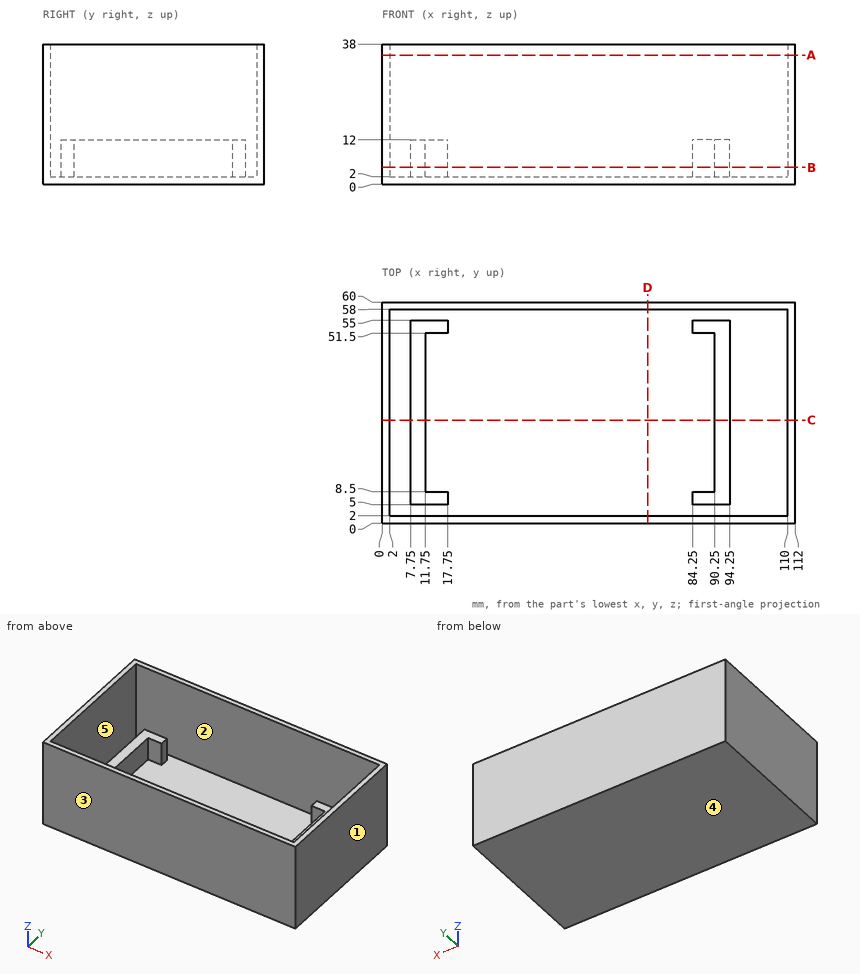
Can you work these out from the drawing? Everything is in mm from the part's minimum corner. A direction names the side the tool comes from. Round coordinates to 2 decimals unless told otherwise and drop trailing zeros. Write each loop counter-clockwise with the first axis right and the second up, starting at its lowest first coordinate (ties: lowest second). Pieces come first, ordered by that corner, then holes. Notation, with made-up numbers: (81.25, -28) - (86.25, -28) arc R9 ccw to (86.25, -21) - close; hole circle Ø2 at (69.25, 65). An arc over 180 degrees is marked (long way). Write each question's results on one line, items separated by ' | '. Start each with the question number.
1) Suppose I cut it at C-C (y = 28). List the corners of the cut face in (x, z) for me.
2) Please list where these lines run through material, in increasing order: line 1 (X direction, y = 32, z = 5); line 2 (X direction, y = 52.5, z = 4.5); line 3 (X direction, y = 44, z = 21).
3) Suppose I cut it at B-B (z = 4.5). List the corners of the cut face in (x, y) for me.
4) Suppose I cut it at A-A (z = 35). List the corners of the cut face in (x, y) for me.
5) We'd pull the mould along Y, two halves only. Please class the marked faces 3, 4 and 5: released by +Y, released by -Y, zero draft, split by the parting line, or undercut.
6) Which directions (+Z, -Z, +X, -X, +Y, -Y) give clear straight access to the entire face, cutting with the end or side of a thin tool? Please do the marked faces 1 and 2.
7) Suppose I cut it at D-D (x = 72). List the corners of the cut face in (y, z) for me.
8) For pin 1 Ø1 at (y, z) = (53, 8.5) entering from -X; pin 2 Ø8 at (x, y) = (12.5, 19) entering from +Z; pin 3 Ø1.5 at (x, y) = (84.5, 34.5) entering from +Z, each with a flat end and sliding along its axis, tell me the tip position at first contact or that it passes through.
Here are the results:
1) outline: (0, 0) - (112, 0) - (112, 38) - (110, 38) - (110, 2) - (94.25, 2) - (94.25, 12) - (90.25, 12) - (90.25, 2) - (11.75, 2) - (11.75, 12) - (7.75, 12) - (7.75, 2) - (2, 2) - (2, 38) - (0, 38) - close
2) line 1: x = 0 to 2, 7.75 to 11.75, 90.25 to 94.25, 110 to 112 | line 2: x = 0 to 2, 7.75 to 17.75, 84.25 to 94.25, 110 to 112 | line 3: x = 0 to 2, 110 to 112
3) outline: (0, 0) - (112, 0) - (112, 60) - (0, 60) - close; (7.75, 5) - (17.75, 5) - (17.75, 8.5) - (11.75, 8.5) - (11.75, 51.5) - (17.75, 51.5) - (17.75, 55) - (7.75, 55) - close; (84.25, 5) - (94.25, 5) - (94.25, 55) - (84.25, 55) - (84.25, 51.5) - (90.25, 51.5) - (90.25, 8.5) - (84.25, 8.5) - close; hole (2, 2) - (110, 2) - (110, 58) - (2, 58) - close
4) outline: (0, 0) - (112, 0) - (112, 60) - (0, 60) - close; hole (2, 2) - (110, 2) - (110, 58) - (2, 58) - close
5) face 3: released by -Y | face 4: zero draft | face 5: undercut
6) face 1: +Z, -Z, +X, +Y, -Y | face 2: +Z
7) outline: (0, 0) - (60, 0) - (60, 38) - (58, 38) - (58, 2) - (2, 2) - (2, 38) - (0, 38) - close
8) pin 1: stops at x = 0 | pin 2: stops at z = 12 | pin 3: stops at z = 2
